```python
from build123d import *

# Parameters (mm, degrees)
BOSS_EXTRUDE1_DEPTH = 1


with BuildPart() as part:
    # Sketch1 → Boss-Extrude1 (new body)
    with BuildSketch(Plane(origin=(0, 0, 0), x_dir=(1, 0, 0), z_dir=(0, 1, 0))):
        with BuildLine():
            Line((2.5, 18.255136264), (2.5, 18))
            ThreePointArc((2.5, 18), (2.353553391, 17.646446609), (2, 17.5))
            Line((2, 17.5), (-2, 17.5))
            ThreePointArc((-2, 17.5), (-2.353553391, 17.646446609), (-2.5, 18))
            Line((-2.5, 18), (-2.5, 18.605106826))
            ThreePointArc((-2.5, 18.605106826), (-2.569127315, 18.756342868), (-2.728723404, 18.803033494))
            ThreePointArc((-2.728723404, 18.803033494), (-0.178274953, -18.999163614), (3.081081081, 18.748518325))
            ThreePointArc((3.081081081, 18.748518325), (2.67638027, 18.636279636), (2.5, 18.255136264))
        make_face()
    extrude(amount=BOSS_EXTRUDE1_DEPTH)


solid = part.part
```
Can you work these out from the model? Positions are in its coordinate system, mm. Round coordinates to 2 decimals unless told otherwise and drop trailing zeros. Loops run counter-clockwise (first coordinate to the right, second up) from the corner with the lowest first, then second, coordinate; pieces in that order, holes last. Notation, with made-up numbers: M 57,-11 L 104,-11 A15 ccw 104,8 Z; hole C -39,-4 d5. An arc over 180 degrees is marked long. Answer in a Markdown table with one row per item.
1. Please list where these lines run through material, in increasing order: line 1 (X direction, y = 0.5, z = 0); line 2 (Z direction, x = 10, y = 0.55); line 3 (Z direction, x = 8.5, y = 0.5). Write a range as from..to.
Established:
| item | result |
|---|---|
| line 1 | -19..19 |
| line 2 | -16.16..16.16 |
| line 3 | -16.99..16.99 |
2. Thinking about a two-plate mould opening in X: for faces 1 (the face through (0, 1, 0)), 2 (the face through (0, 0.5, -17.5)), 3 (the face through (-0.973, 0.493, 18.975)), which applies, pulls with the +X half, pulls with the -X half, needs draft (parallel to the pull), parting line crosses it, or undercut?
Established:
| item | result |
|---|---|
| face 1 | needs draft |
| face 2 | undercut |
| face 3 | parting line crosses it |
3. If we section it at A-A, the plane y = 0.3: Please give me the cut outline in (x, z).
Established:
| item | result |
|---|---|
| outline | M -2.73,-18.8 A0.2 ccw -2.5,-18.61 L -2.5,-18 A0.5 cw -2,-17.5 L 2,-17.5 A0.5 cw 2.5,-18 L 2.5,-18.26 A0.5 ccw 3.08,-18.75 A19 ccw long Z |
4. If we section it at B-B, the plane x = 0: Please give me the cut outline in (y, z), plus the area to 3 significant figures.
Established:
| item | result |
|---|---|
| outline | M 0,-17.5 L 1,-17.5 L 1,19 L 0,19 Z |
| area | 36.5 mm² |
5. If we section it at C-C, the plane z = -14: Please give me the cut outline in (x, y).
Established:
| item | result |
|---|---|
| outline | M -12.85,0 L 12.85,0 L 12.85,1 L -12.85,1 Z |
